Source: CAD feature listing. Evaluate the final solid. Frame: model axes, mm. Face numbers are marked on the shaded views. A direction names the side the tool comes from. Coordinates: 2 decimals unless noted, no trailing zeros. Loops run counter-clockwise (first coordinate to the right, second up) from the corner with the lowest first, then second, coordinate; pieces in that order, holes last. Notation, with made-up numbers: (-40, 50) - (10, 50) arc R29 cw to (10, 82) - close; hole circle Ø6 at (-28.5, -4). An arc over 180 degrees is marked (long way). Use one line per item in the form item = value. Start each with the question number.
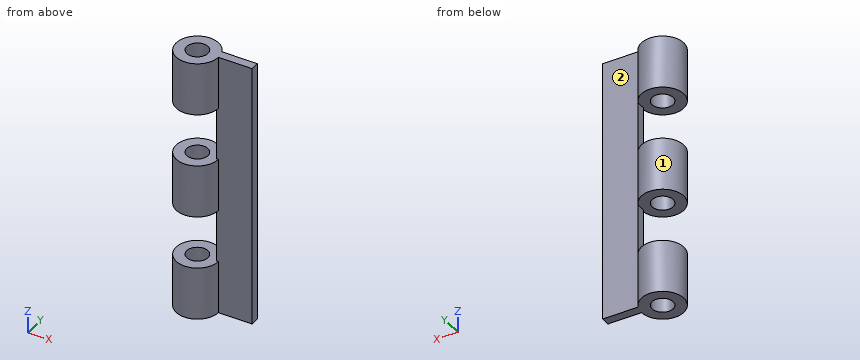
from build123d import *

# Parameters (mm, degrees)
SKETCH1_W           = 20
SKETCH1_H           = 150
BOSS_EXTRUDE1_DEPTH = 2.5
SKETCH5_R           = 12
SKETCH5_R_2         = 6
BOSS_EXTRUDE2_DEPTH = 30
LPATTERN1_COUNT     = 3
LPATTERN1_PITCH     = 60


with BuildPart() as part:
    # Sketch1 → Boss-Extrude1 (new body, symmetric)
    with BuildSketch(Plane(origin=(0, 0, 0), x_dir=(1, 0, 0), z_dir=(0, 1, 0))):
        Rectangle(SKETCH1_W, SKETCH1_H)
    extrude(amount=BOSS_EXTRUDE1_DEPTH, both=True)

    # Sketch5 → Boss-Extrude2 (add)
    with BuildSketch(Plane.XY.offset(75)):
        with Locations((-21.009649651, -2.273637457)):
            Circle(SKETCH5_R)
        with Locations((-21.009649651, -2.273637457)):
            Circle(SKETCH5_R_2, mode=Mode.SUBTRACT)
    boss_extrude2 = extrude(amount=-BOSS_EXTRUDE2_DEPTH)

    # LPattern1: Boss-Extrude2 ×3
    with Locations(*[(0, 0, -i * LPATTERN1_PITCH) for i in range(1, LPATTERN1_COUNT)]):
        add(boss_extrude2)


solid = part.part
(1) Material intervals for line 1 (Z direction, x = -29.5, y = -4.75); line 2 (Y direction, x = -18, z = 46.5); line 3 (X direction, y = -2.25, z = 59), sorted ascending.
(2) Access query for the marked faces 1 and 2. Directions: +Z, -Z, +X, -X, +Y, -Y. A direction counts if a zero-diameter tool reaches every point of the face in a straight line with its end or side. Return the directions, or none.
(3) Cut plane A-A, the plane x = -29. Output: boundary loops of the cut face in (y, z).
(4) Cut plane B-B, the plane y = 7.25. Output: boundary loops of the cut face in (x, z).
(5) Cut plane D-D, the plane z = 48. Output: boundary loops of the cut face in (x, y).
(6) Contact query for flat-ended pins moving along their axis: pin 1 (10 mm diameter, centred on x = 3, z = 50, fed in from -Y); pin 2 (22 mm diameter, centred on x = 4, z = 23, fed in from +Y); pin 3 (1.5 mm diameter, centred on x = -1.5, y = 4, fed in from -Z); pin 4 (4 mm diameter, centred on y = 0.5, z = 24.5, fed in from -X). Output: stop coordinate, or through.
(7) Cut plane C-C, the plane y = -5. Output: boundary loops of the cut face in (x, z).
Recorded:
q1.line_1 = -75 to -45, -15 to 15, 45 to 75
q1.line_2 = -13.89 to -7.46, 2.92 to 9.34
q1.line_3 = -33.01 to -27.01, -15.01 to 10
q2.face_1 = +Z, -Z
q2.face_2 = +Z, -Z, +X, +Y
q3.outline = (-11.23, -75) - (6.68, -75) - (6.68, -45) - (-11.23, -45) - close; (-11.23, -15) - (6.68, -15) - (6.68, 15) - (-11.23, 15) - close; (-11.23, 45) - (6.68, 45) - (6.68, 75) - (-11.23, 75) - close
q4.outline = (-28.31, -75) - (-13.71, -75) - (-13.71, -45) - (-28.31, -45) - close; (-28.31, -15) - (-13.71, -15) - (-13.71, 15) - (-28.31, 15) - close; (-28.31, 45) - (-13.71, 45) - (-13.71, 75) - (-28.31, 75) - close
q5.outline = (-10, 2.5) arc R12 ccw (long way) to (-9.01, -2.5) - (10, -2.5) - (10, 2.5) - close; hole circle Ø12 at (-21.01, -2.27)
q6.pin_1 = -2.5
q6.pin_2 = 2.5
q6.pin_3 = through
q6.pin_4 = -10
q7.outline = (-32.7, -75) - (-26.35, -75) - (-26.35, -45) - (-32.7, -45) - close; (-32.7, -15) - (-26.35, -15) - (-26.35, 15) - (-32.7, 15) - close; (-32.7, 45) - (-26.35, 45) - (-26.35, 75) - (-32.7, 75) - close; (-15.66, -75) - (-9.32, -75) - (-9.32, -45) - (-15.66, -45) - close; (-15.66, -15) - (-9.32, -15) - (-9.32, 15) - (-15.66, 15) - close; (-15.66, 45) - (-9.32, 45) - (-9.32, 75) - (-15.66, 75) - close
